```python
from build123d import *

# Parameters (mm, degrees)
SKETCH1_W           = 50
SKETCH1_H           = 700
BOSS_EXTRUDE1_DEPTH = 5
SKETCH3_R           = 2
CUT_EXTRUDE1_DEPTH  = 6
SKETCH5_W           = 10
SKETCH5_H           = 700
CUT_EXTRUDE2_DEPTH  = 2.5
SKETCH6_R           = 3
CUT_EXTRUDE3_DEPTH  = 6


with BuildPart() as part:
    # Sketch1 → Boss-Extrude1 (new body)
    with BuildSketch(Plane(origin=(0, 0, 0), x_dir=(1, 0, 0), z_dir=(0, 1, 0))):
        with Locations((25, 350)):
            Rectangle(SKETCH1_W, SKETCH1_H)
    extrude(amount=BOSS_EXTRUDE1_DEPTH)

    # Sketch3 → Cut-Extrude1 (cut, through all)
    with BuildSketch(Plane(origin=(0, 5, 0), x_dir=(1, 0, 0), z_dir=(0, 1, 0))):
        with Locations((25, 600)):
            Circle(SKETCH3_R)
        with Locations((25, 350)):
            Circle(SKETCH3_R)
        with Locations((25, 100)):
            Circle(SKETCH3_R)
    extrude(amount=-CUT_EXTRUDE1_DEPTH, mode=Mode.SUBTRACT)

    # Sketch5 → Cut-Extrude2 (cut)
    with BuildSketch(Plane(origin=(0, 5, 0), x_dir=(1, 0, 0), z_dir=(0, 1, 0))):
        with Locations((7, 350)):
            Rectangle(SKETCH5_W, SKETCH5_H)
        with Locations((43, 350)):
            Rectangle(SKETCH5_W, SKETCH5_H)
    extrude(amount=-CUT_EXTRUDE2_DEPTH, mode=Mode.SUBTRACT)

    # Sketch6 → Cut-Extrude3 (cut, through all)
    with BuildSketch(Plane(origin=(0, 5, 0), x_dir=(1, 0, 0), z_dir=(0, 1, 0))):
        with Locations((43, 25)):
            Circle(SKETCH6_R)
        with Locations((7, 25)):
            Circle(SKETCH6_R)
        with Locations((43, 675)):
            Circle(SKETCH6_R)
        with Locations((7, 675)):
            Circle(SKETCH6_R)
    extrude(amount=-CUT_EXTRUDE3_DEPTH, mode=Mode.SUBTRACT)


solid = part.part
```
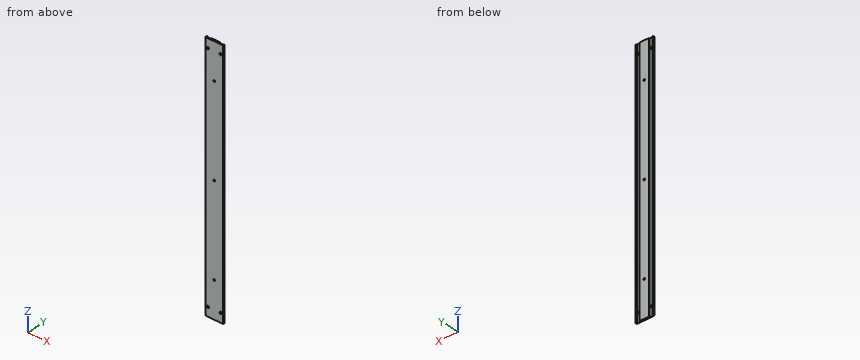
Here's how the part is built. I have some questions about the finished solid (model axes, mm). Coordinates: 2 decimals unless noted, no trailing zeros. Loops run counter-clockwise (first coordinate to the right, second up) from the corner with the lowest first, then second, coordinate; pieces in that order, holes last. Notation, with made-up numbers: (14, 20.5) - (19, 20.5) arc R29 cw to (19, 59.5) - close; hole circle Ø8 at (85.25, 82.25). An arc over 180 degrees is marked (long way). Answer as CSV lines item,"result".
Q1. If I drill on L1, parallel to X at y = 3.7, z = -546; L2, parallel to Z at x = 25, y = 1.85; L3, parallel to Z at x = 43, y = 0.8, over which ranges is the centre line in solid material (lowest first)? Write a range as [from, to].
Response:
L1,"[0, 2], [12, 38], [48, 50]"
L2,"[-700, -602], [-598, -352], [-348, -102], [-98, 0]"
L3,"[-700, -678], [-672, -28], [-22, 0]"
Q2. For pin 1 (3 mm diameter, centred on x = 41, z = -459, fed in from +Y), with a flat end and sliding along its axis, tell me the tip position at first contact or that it passes through.
Response:
pin 1,"y = 2.5"
Q3. If we section it at A-A, the plane z = -191: Write out the boundary of the cut face in (x, y).
Response:
outline,"(0, 0) - (50, 0) - (50, 5) - (48, 5) - (48, 2.5) - (38, 2.5) - (38, 5) - (12, 5) - (12, 2.5) - (2, 2.5) - (2, 5) - (0, 5) - close"
